CAD build for the part. Positions are in the model's coordinates, mm. A direction names the side the tool comes from. Round coordinates to 2 decimals unless told otherwise and drop trailing zeros. Write each loop counter-clockwise with the first axis right and the second up, starting at its lowest first coordinate (ties: lowest second). Pieces come first, ordered by that corner, then holes. Notation, with made-up numbers: (-39, -14.75) - (-23, -14.75) arc R16 cw to (-23, 3.25) - close; hole circle Ø8 at (17.5, 66). An arc over 180 degrees is marked (long way). Use one line per item in the form item = value. Start each with the question number.
Item 1: Band-saw the part on C-C, the plane x = -8.5. List the corners of the cut face in (y, z).
Item 2: Pin check, flat tips, straight feed: pin 1 (6 mm diameter, centred on y = 102.5, z = 10.5, fed in from -X); pin 2 (4 mm diameter, centred on y = 121, z = 8, fed in from +X); pin 3 (4 mm diameter, centred on x = -1.5, z = 1.5, fed in from -Y); pin 4 (3 mm diameter, centred on x = -88.5, y = 91, fed in from +Z). Stop position of each tip, or through.
Item 3: Band-saw the part on A-A, the plane x = -47. List the corners of the cut face in (y, z).
Item 4: Band-saw the part on B-B, the plane z = 12.5. List the corners of the cut face in (x, y).
Item 5: Drill centre lines: L1, parallel to Y at x = -47, z = 1.85; L2, parallel to X at y = 121.7, z = 8; L3, parallel to Y at x = -67, z = 5.25. Where is each one in solid material? Low to high.
Item 6: Pull direction X, two halves, no side cores. Call faces 1 (the cylindrical face through (-67, 122, 8)), 2 (the flat face through (-93, 5, 10)), 3 (the flat face through (-95, 3.8, 3.8)): +X half, -X half, draft (parallel to the pull), parting line (faces both ways), or undercut.
Item 7: Tool access for faces 4 (the flat face through (-88, 10, 4)), 5 (the flat face through (-77, 122, 9)), 6 (the flat face through (-93, 115, 7)): list every direction of +Z, -Z, +X, -X, +Y, -Y with a clear straight run to the whole face (end or side of a thin tool).
Item 8: Band-saw the part on D-D, the plane y = 65. List the corners of the cut face in (x, z).
from build123d import *

# Parameters (mm, degrees)
SKETCH1_W           = 90
SKETCH1_H           = 125
BOSS_EXTRUDE1_DEPTH = 5
SKETCH2_W           = 5
SKETCH2_H           = 105
BOSS_EXTRUDE2_DEPTH = 5
SKETCH3_W           = 5
SKETCH3_H           = 10
BOSS_EXTRUDE3_DEPTH = 5
SKETCH4_W           = 5
SKETCH4_H           = 10
CUT_EXTRUDE1_DEPTH  = 3
SKETCH5_R           = 1.5
CUT_EXTRUDE2_DEPTH  = 15
CUT_EXTRUDE3_START  = -15
SKETCH6_R           = 1.5
CUT_EXTRUDE3_DEPTH  = 15
SKETCH7_W           = 53
SKETCH7_H           = 5
SKETCH7_W_2         = 70
BOSS_EXTRUDE4_DEPTH = 9
CUT_EXTRUDE4_REACH  = 162.689
SKETCH8_R           = 1.75
SKETCH9_R           = 1.5
CUT_EXTRUDE5_DEPTH  = 5
SKETCH10_R          = 2
CUT_EXTRUDE6_DEPTH  = 5
SKETCH11_W          = 5
SKETCH11_H          = 105
BOSS_EXTRUDE5_DEPTH = 5


with BuildPart() as part:
    # Sketch1 → Boss-Extrude1 (new body)
    with BuildSketch(Plane.XY):
        with Locations((-50, 62.5)):
            Rectangle(SKETCH1_W, SKETCH1_H)
    extrude(amount=BOSS_EXTRUDE1_DEPTH)

    # Sketch2 → Boss-Extrude2 (add)
    with BuildSketch(Plane.ZY.offset(95)):
        with Locations((2.5, 62.5)):
            Rectangle(SKETCH2_W, SKETCH2_H)
    extrude(amount=BOSS_EXTRUDE2_DEPTH)

    # Sketch3 → Boss-Extrude3 (add)
    with BuildSketch(Plane.XY.offset(5)):
        with Locations((-7.5, 120)):
            Rectangle(SKETCH3_W, SKETCH3_H)
        with Locations((-92.5, 120)):
            Rectangle(SKETCH3_W, SKETCH3_H)
        with Locations((-7.5, 5)):
            Rectangle(SKETCH3_W, SKETCH3_H)
        with Locations((-92.5, 5)):
            Rectangle(SKETCH3_W, SKETCH3_H)
    extrude(amount=BOSS_EXTRUDE3_DEPTH)

    # Sketch4 → Cut-Extrude1 (cut)
    with BuildSketch(Plane.XY.offset(5)):
        with Locations((-87.5, 120)):
            Rectangle(SKETCH4_W, SKETCH4_H)
        with Locations((-12.5, 120)):
            Rectangle(SKETCH4_W, SKETCH4_H)
        with Locations((-12.5, 5)):
            Rectangle(SKETCH4_W, SKETCH4_H)
        with Locations((-87.5, 5)):
            Rectangle(SKETCH4_W, SKETCH4_H)
    extrude(amount=-CUT_EXTRUDE1_DEPTH, mode=Mode.SUBTRACT)

    # Sketch5 → Cut-Extrude2 (cut)
    with BuildSketch(Plane(origin=(0, 0, 0), x_dir=(0, 0, -1), z_dir=(1, 0, 0))):
        with Locations(Location((-5, 5, 0), (0, 0, 90))):
            Circle(SKETCH5_R)
        with Locations(Location((-5, 120, 0), (0, 0, 90))):
            Circle(SKETCH5_R)
    extrude(amount=-CUT_EXTRUDE2_DEPTH, mode=Mode.SUBTRACT)

    # Sketch6 → Cut-Extrude3 (cut)
    with BuildSketch(Plane.ZY.offset(100).offset(CUT_EXTRUDE3_START)):
        with Locations(Location((5, 5, 0), (0, 0, 90))):
            Circle(SKETCH6_R)
        with Locations(Location((5, 120, 0), (0, 0, 90))):
            Circle(SKETCH6_R)
    extrude(amount=CUT_EXTRUDE3_DEPTH, mode=Mode.SUBTRACT)

    # Sketch7 → Boss-Extrude4 (add)
    with BuildSketch(Plane.XY.offset(5)):
        with Locations((-50.5, 122.5)):
            Rectangle(SKETCH7_W, SKETCH7_H)
        with Locations((-50, 2.5)):
            Rectangle(SKETCH7_W_2, SKETCH7_H)
    extrude(amount=BOSS_EXTRUDE4_DEPTH)

    # Cut-Extrude4: up to this face of the body (flat: up to its plane)
    cut_extrude4_end = Plane(part.part.faces().sort_by_distance((-50.251847941, 125, 6.258183738))[0])
    # Sketch8 → Cut-Extrude4 (cut, up to the picked face)
    with BuildSketch(Plane.XZ, mode=Mode.PRIVATE) as cut_extrude4_sk1:
        with Locations(Location((-65.25, 8, 0), (0, 0, 270))):
            Circle(SKETCH8_R)
    cut_extrude4_tool1 = split(extrude(cut_extrude4_sk1.sketch, amount=-CUT_EXTRUDE4_REACH, mode=Mode.PRIVATE), bisect_by=cut_extrude4_end, keep=Keep.BOTH, mode=Mode.PRIVATE)
    # Sketch8 → Cut-Extrude4 (cut, up to the picked face)
    with BuildSketch(Plane.XZ, mode=Mode.PRIVATE) as cut_extrude4_sk2:
        with Locations(Location((-50.25, 8, 0), (0, 0, 270))):
            Circle(SKETCH8_R)
    cut_extrude4_tool2 = split(extrude(cut_extrude4_sk2.sketch, amount=-CUT_EXTRUDE4_REACH, mode=Mode.PRIVATE), bisect_by=cut_extrude4_end, keep=Keep.BOTH, mode=Mode.PRIVATE)
    # Sketch8 → Cut-Extrude4 (cut, up to the picked face)
    with BuildSketch(Plane.XZ, mode=Mode.PRIVATE) as cut_extrude4_sk3:
        with Locations(Location((-35.25, 8, 0), (0, 0, 270))):
            Circle(SKETCH8_R)
    cut_extrude4_tool3 = split(extrude(cut_extrude4_sk3.sketch, amount=-CUT_EXTRUDE4_REACH, mode=Mode.PRIVATE), bisect_by=cut_extrude4_end, keep=Keep.BOTH, mode=Mode.PRIVATE)
    add(cut_extrude4_tool1.solids().sort_by(Axis((-65.25, 0, 8), (0, 1, 0)))[0], mode=Mode.SUBTRACT)
    add(cut_extrude4_tool2.solids().sort_by(Axis((-50.25, 0, 8), (0, 1, 0)))[0], mode=Mode.SUBTRACT)
    add(cut_extrude4_tool3.solids().sort_by(Axis((-35.25, 0, 8), (0, 1, 0)))[0], mode=Mode.SUBTRACT)

    # Sketch9 → Cut-Extrude5 (cut)
    with BuildSketch(Plane.XY.offset(5)):
        with Locations((-47, 101)):
            Circle(SKETCH9_R)
        with Locations((-90, 101)):
            Circle(SKETCH9_R)
        with Locations((-90, 58)):
            Circle(SKETCH9_R)
        with Locations((-47, 58)):
            Circle(SKETCH9_R)
    extrude(amount=-CUT_EXTRUDE5_DEPTH, mode=Mode.SUBTRACT)

    # Sketch10 → Cut-Extrude6 (cut)
    with BuildSketch(Plane.XY.offset(5)):
        with Locations((-85, 33)):
            Circle(SKETCH10_R)
        with Locations((-24, 33)):
            Circle(SKETCH10_R)
    extrude(amount=-CUT_EXTRUDE6_DEPTH, mode=Mode.SUBTRACT)

    # Sketch11 → Boss-Extrude5 (add)
    with BuildSketch(Plane(origin=(-5, 0, 0), x_dir=(0, 0, -1), z_dir=(1, 0, 0))):
        with Locations((-2.5, 62.5)):
            Rectangle(SKETCH11_W, SKETCH11_H)
    extrude(amount=BOSS_EXTRUDE5_DEPTH)


solid = part.part
Determined:
q1.outline = (0, 0) - (125, 0) - (125, 10) - (115, 10) - (115, 5) - (10, 5) - (10, 10) - (0, 10) - close; hole circle Ø3 at (5, 5); hole circle Ø3 at (120, 5)
q2.pin_1 = through
q2.pin_2 = -5
q2.pin_3 = 10
q2.pin_4 = 5
q3.outline = (0, 0) - (56.5, 0) - (56.5, 5) - (5, 5) - (5, 14) - (0, 14) - close; (59.5, 0) - (99.5, 0) - (99.5, 5) - (59.5, 5) - close; (102.5, 0) - (125, 0) - (125, 14) - (120, 14) - (120, 5) - (102.5, 5) - close
q4.outline = (-85, 0) - (-15, 0) - (-15, 5) - (-85, 5) - close; (-77, 120) - (-24, 120) - (-24, 125) - (-77, 125) - close
q5.L1 = 0 to 56.5, 59.5 to 99.5, 102.5 to 125
q5.L2 = -95 to -90, -77 to -67, -63.5 to -52, -48.5 to -37, -33.5 to -24, -10 to -5
q5.L3 = 0 to 5, 120 to 125
q6.face_1 = undercut
q6.face_2 = draft
q6.face_3 = -X half
q7.face_4 = +Z, -Y
q7.face_5 = +Z, +Y
q7.face_6 = +Z, +X, -X
q8.outline = (-100, 0) - (0, 0) - (0, 5) - (-100, 5) - close
